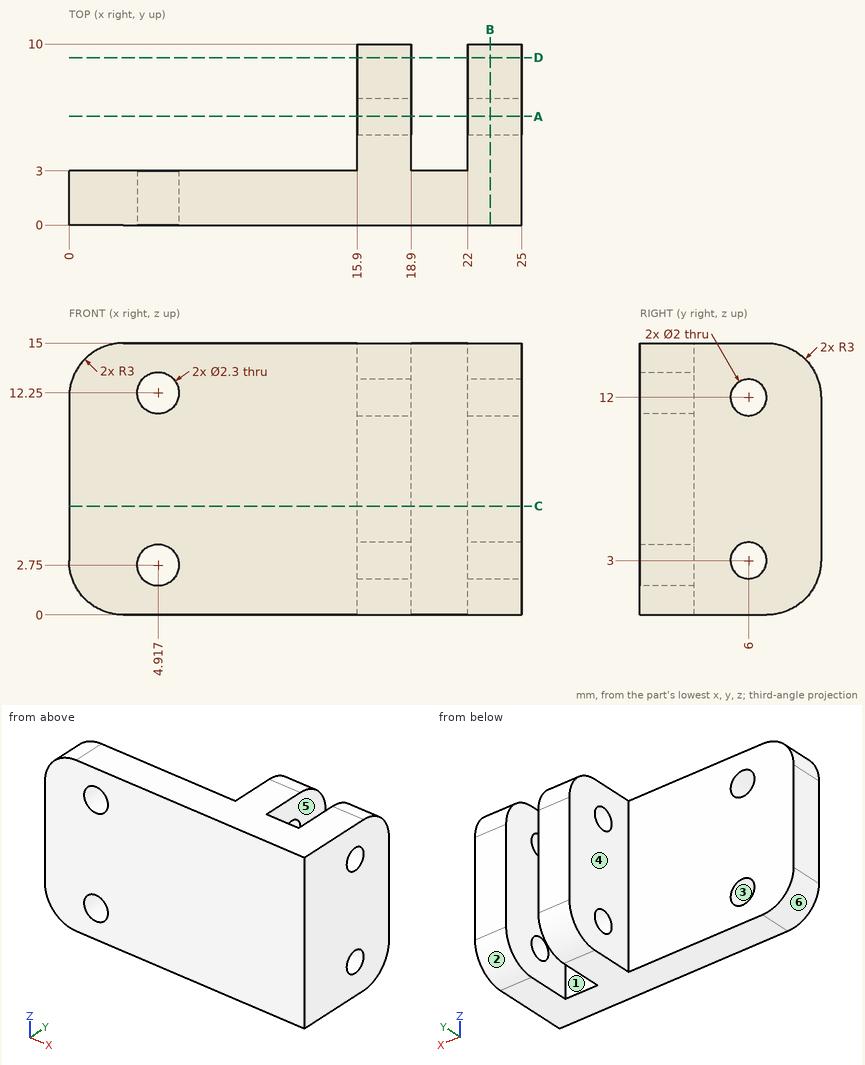
Can you work these out from the drawing? Everything is in mm from the part's minimum corner. A direction names the side the tool comes from. Coordinates: 2 decimals unless noted, no trailing zeros. Write each loop counter-clockwise with the first axis right and the second up, starting at its lowest first coordinate (ties: lowest second). Pieces come first, ordered by that corner, then holes. Notation, with made-up numbers: (63.5, 26.25) - (89.5, 26.25) arc R20 ccw to (89.5, 38.25) - close; hole circle Ø8 at (83.25, 10.5). An arc over 180 degrees is marked (long way). Use a Markdown table: item, result.
Q1. I'm going to push flat-ended pins straight in: pin 1 Ø3 at (y, z) = (6, 12) entering from -X; pin 2 Ø1.2 at (y, z) = (6, 12) entering from -X; pin 3 Ø4.5 at (x, z) = (4.5, 6) entering from +Y. Where does each tip first touch, or does it pass through?
Geometry check:
| item | result |
|---|---|
| pin 1 | stops at x = 15.9 |
| pin 2 | passes through |
| pin 3 | stops at y = 3 |
Q2. Thinking about a two-plate mould opening in Z: for the marked faces 1, 2 and 3, which applies, +Z half, -Z half, draft (parallel to the pull), parting line (faces both ways), or undercut?
Geometry check:
| item | result |
|---|---|
| face 1 | draft |
| face 2 | -Z half |
| face 3 | undercut |
Q3. Which directions (+Z, -Z, +X, -X, +Y, -Y) give clear straight access to the entire face, cutting with the end or side of a thin tool? Please do the marked faces 4, 5 and 6.
Geometry check:
| item | result |
|---|---|
| face 4 | +Z, -Z, -X, +Y |
| face 5 | +Z, -Z, +Y |
| face 6 | -Z, -X, +Y, -Y |
Q4. Imagine slicing it at D-D (y = 9.25). List the corners of the cut face in (x, z) for me (1 decimal).
Geometry check:
| item | result |
|---|---|
| outline | (15.9, 1) - (18.9, 1) - (18.9, 14) - (15.9, 14) - close; (22, 1) - (25, 1) - (25, 14) - (22, 14) - close |
Q5. Please list where these lines run through material, in increasing order: L1, parallel to Z at x = 23.95, y = 6; L2, parallel to X at y = 5.5, z = 10.25; L3, parallel to Y at x = 18.2, z = 12.
Geometry check:
| item | result |
|---|---|
| L1 | z = 0 to 2, 4 to 11, 13 to 15 |
| L2 | x = 15.9 to 18.9, 22 to 25 |
| L3 | y = 0 to 5, 7 to 10 |
Q6. Imagine slicing it at C-C (z = 6). List the corners of the cut face in (x, y) for me.
Geometry check:
| item | result |
|---|---|
| outline | (0, 0) - (25, 0) - (25, 10) - (22, 10) - (22, 3) - (18.9, 3) - (18.9, 10) - (15.9, 10) - (15.9, 3) - (0, 3) - close |
Q7. Imagine slicing it at A-A (y = 6). List the corners of the cut face in (x, z) for me.
Geometry check:
| item | result |
|---|---|
| outline | (15.9, 0) - (18.9, 0) - (18.9, 2) - (15.9, 2) - close; (15.9, 4) - (18.9, 4) - (18.9, 11) - (15.9, 11) - close; (15.9, 13) - (18.9, 13) - (18.9, 15) - (15.9, 15) - close; (22, 0) - (25, 0) - (25, 2) - (22, 2) - close; (22, 4) - (25, 4) - (25, 11) - (22, 11) - close; (22, 13) - (25, 13) - (25, 15) - (22, 15) - close |
Q8. Imagine slicing it at B-B (x = 23.25). List the corners of the cut face in (y, z) for me, and give its area (3 significant figures).
Geometry check:
| item | result |
|---|---|
| outline | (0, 0) - (7, 0) arc R3 ccw to (10, 3) - (10, 12) arc R3 ccw to (7, 15) - (0, 15) - close; hole circle Ø2 at (6, 3); hole circle Ø2 at (6, 12) |
| area | 140 mm2 |
